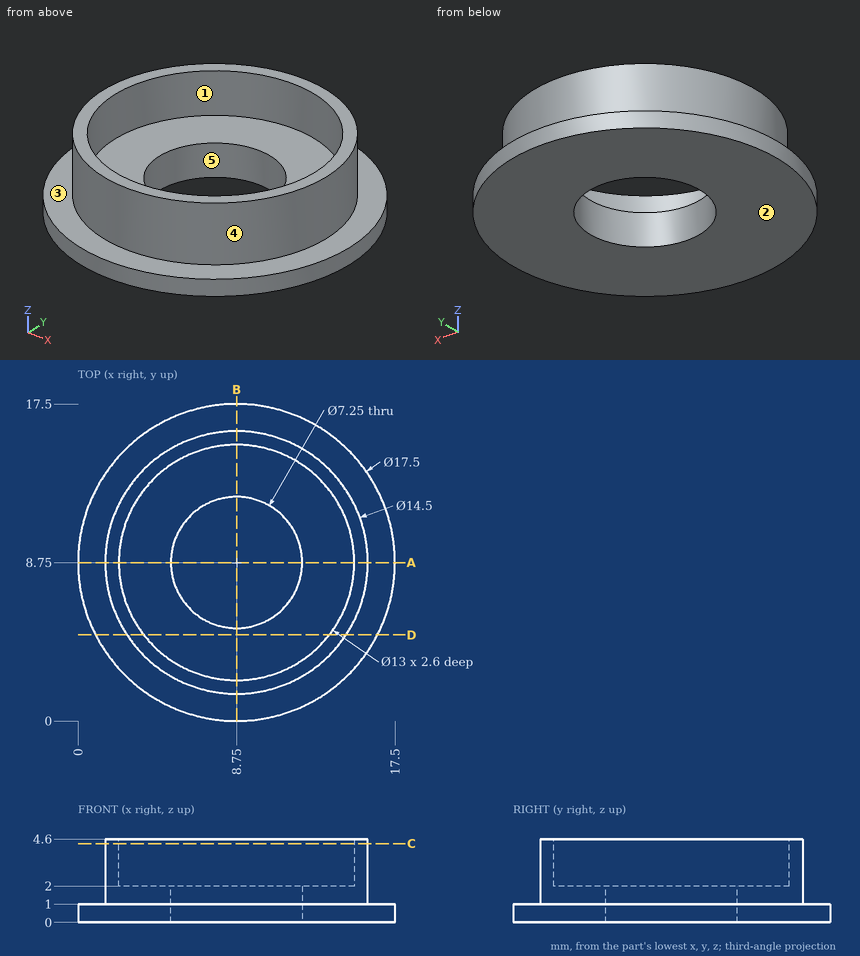
Part print with two shaded views. Sizes in mm from the minimum x, y, z corner. A direction names the side the tool comes from. Round coordinates to 2 decimals unless told otherwise and drop trailing zeros. Loops run counter-clockwise (first coordinate to the right, second up) from the corner with the lowest first, then second, coordinate; pieces in that order, holes last. Notation, with made-up numbers: (-29, 25.5) - (-5, 25.5) arc R21 cw to (-5, 59.5) - close; hole circle Ø9 at (15.5, 53.5). An arc over 180 degrees is marked (long way). Answer as a JSON object with one key per item and string values.
Item 1: Band-saw the part on D-D on y = 4.75. List the corners of the cut face in (x, z).
Output:
{"outline": "(0.97, 0) - (16.53, 0) - (16.53, 1) - (14.8, 1) - (14.8, 4.6) - (13.87, 4.6) - (13.87, 2) - (3.63, 2) - (3.63, 4.6) - (2.7, 4.6) - (2.7, 1) - (0.97, 1) - close"}
Item 2: Band-saw the part on C-C on z = 4.35. List the corners of the cut face in (x, y).
Output:
{"outline": "circle Ø14.5 at (8.75, 8.75); hole circle Ø13 at (8.75, 8.75)"}
Item 3: Wall check: L1, parallel to Y at x = 8.75, z = 3.05; L2, parallel to Z at x = 15.75, y = 5.25; L3, parallel to Y at x = 8.75, z = 1.3 (3 decimals). Give the ranges that are in metal, low to high.
Output:
{"L1": "1.5 to 2.25, 15.25 to 16", "L2": "0 to 1", "L3": "1.5 to 5.125, 12.375 to 16"}
Item 4: Pin check, flat tips, straight feed: pin 1 (1 mm diameter, centred on x = 15.5, z = 2, fed in from -Y); pin 2 (1 mm diameter, centred on x = 7, z = 3, fed in from +Y); pin 3 (2 mm diameter, centred on y = 9, z = 3, fed in from -X); pin 4 (6 mm diameter, centred on x = 8.75, y = 8.75, fed in from -Z). Stop position of each tip, or through.
Output:
{"pin 1": "y = 5.08", "pin 2": "y = 15.89", "pin 3": "x = 1.5", "pin 4": "through"}
Item 5: Pull direction X, two halves, no side cores. Call the marked faces 3, 4 and 5: pulls with the +X half, pulls with the -X half, needs draft (parallel to the pull), parting line crosses it, or undercut.
Output:
{"face 3": "needs draft", "face 4": "parting line crosses it", "face 5": "undercut"}
Item 6: Band-saw the part on A-A on y = 8.75. List the corners of the cut face in (x, z) (3 decimals).
Output:
{"outline": "(0, 0) - (5.125, 0) - (5.125, 2) - (2.25, 2) - (2.25, 4.6) - (1.5, 4.6) - (1.5, 1) - (0, 1) - close; (12.375, 0) - (17.5, 0) - (17.5, 1) - (16, 1) - (16, 4.6) - (15.25, 4.6) - (15.25, 2) - (12.375, 2) - close"}
Item 7: Tool access for the marked faces 1 and 2: list every direction of +Z, -Z, +X, -X, +Y, -Y with a clear straight run to the whole face (end or side of a thin tool).
Output:
{"face 1": "+Z", "face 2": "-Z, +X, -X, +Y, -Y"}
